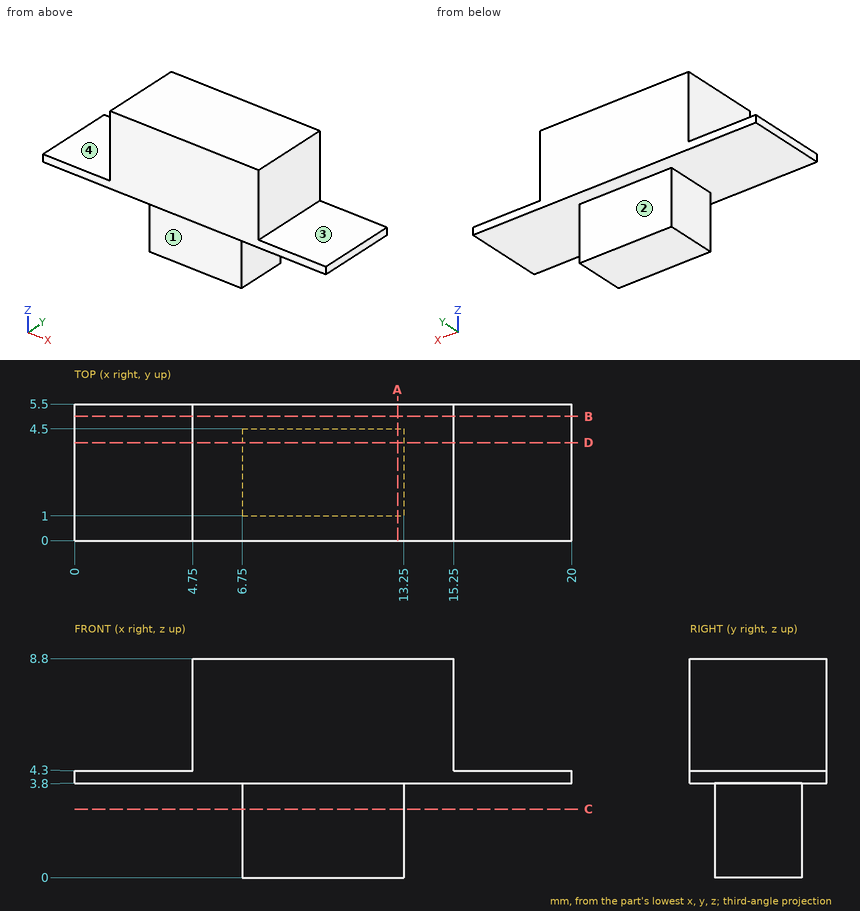
Study the drawing (mm; zero at the part's minimum x, y, z) and answer. A direction names the side the tool comes from. Coordinates: 2 decimals unless noted, no trailing zeros. Order: outer loops, then holes, each group sorted by start corner. A loop starts at its lowest first (then second) coordinate and runs counter-clockwise, first axis right, second up. Notation, with made-up numbers: M 82,51 L 123,51 A21 cw 123,78 Z; hole C 31.5,16.25 d5. An arc over 180 degrees is marked long. Use CSV: the item, a comma, the result in double quotes.
Q1. Section D-D (y = 3.95) is taken. Determine the outline of the cut face in (x, z), then the cut area to 4 significant figures.
Here are the results:
outline,"M 0,3.8 L 6.75,3.8 L 6.75,0 L 13.25,0 L 13.25,3.8 L 20,3.8 L 20,4.3 L 15.25,4.3 L 15.25,8.8 L 4.75,8.8 L 4.75,4.3 L 0,4.3 Z"
area,"81.95 mm2"
Q2. Section C-C (z = 2.75) is taken. Determine the outline of the cut face in (x, y).
Here are the results:
outline,"M 6.75,1 L 13.25,1 L 13.25,4.5 L 6.75,4.5 Z"
Q3. A tool of negligible diameter and unlimited length cuts with its end or side. For the marked faces 1, 2, 3 and 4, from which of +Z, -Z, +X, -X, +Y, -Y can it reach the whole face along a straight path? Write none if from no direction.
Here are the results:
face 1,"-Z, +X, -X, -Y"
face 2,"-Z, +X, -X, +Y"
face 3,"+Z, +X, +Y, -Y"
face 4,"+Z, -X, +Y, -Y"
Q4. Straight lines are drawn through the part: L1, parallel to X at y = 3.7, z = 5.5; L2, parallel to Z at x = 14.5, y = 1.2; L3, parallel to Y at x = 8.75, z = 2. For each, find the intervals that lie inside material, in ascending order.
Here are the results:
L1,"4.75 to 15.25"
L2,"3.8 to 8.8"
L3,"1 to 4.5"
Q5. Given pin 1 Ø1.1 at (x, z) = (10, 2.5) entering from -Y; pin 2 Ø1 at (y, z) = (3.5, 2.5) entering from -X; pin 3 Ø4 at (x, z) = (11, 1) entering from +Y, each flat-ended and moving along its own axis, determine where each tip first touches the part or whether it passes through.
Here are the results:
pin 1,"y = 1"
pin 2,"x = 6.75"
pin 3,"y = 4.5"
Q6. Section B-B (y = 5) is taken. Determine the outline of the cut face in (x, z), then the cut area to 4 significant figures.
Here are the results:
outline,"M 0,3.8 L 20,3.8 L 20,4.3 L 15.25,4.3 L 15.25,8.8 L 4.75,8.8 L 4.75,4.3 L 0,4.3 Z"
area,"57.25 mm2"
Q7. Section A-A (x = 13) is taken. Determine the outline of the cut face in (y, z), then the cut area to 3 significant figures.
Here are the results:
outline,"M 0,3.8 L 1,3.8 L 1,0 L 4.5,0 L 4.5,3.8 L 5.5,3.8 L 5.5,8.8 L 0,8.8 Z"
area,"40.8 mm2"
